Check sheet for the modelled part. Datum: model origin and axes. Units: mm. A direction names the side the tool comes from. Give positions to 0.01 mm unless a question says otherwise; leave off trailing zeros. Write each loop counter-clockwise with the first axis right and the second up, starting at its lowest first coordinate (ties: lowest second). Pieces come first, ordered by that corner, then holes. Notation, with made-up numbers: (23.25, -24.75) -> (69.25, -24.75) arc R19 ccw to (69.25, 3.25) -> close; hole circle Ø1 at (57.5, 22.25). An arc over 180 degrees is marked (long way). Use a Markdown table: item, result. Add a question column.
1. Set-up check for faces 4 (the flat face through (1.15, 8, 1)), 5 (the flat face through (4, -4, 0)): record each of +Z, -Z, +X, -X, +Y, -Y from which the full face is reachable in a straight line by a thin tool's end or side.
2. Cross-section at C-C (z = 3.3). Enter the section's corners in (x, y).
3. Cross-section at A-A (x = 0). Enter the section's corners in (y, z).
4. Gauge pin test, flat ends, axial feed: P1, Ø2, axis at y = 9, z = 2, coming from the +X side; P2, Ø2, axis at x = -10.5, z = 1.5, coming from the +Y side; P3, Ø1, axis at y = -14, z = 3, coming from the +X side; P4, Ø1.2, axis at y = -0.5, z = 1, coming from the -X side. Record the tip position at first contact, or that the pin passes through.
5. Scan lines: probe 1 along Y at (x, z) = (-0.5, 0.75); probe 2 along X at (y, z) = (-10.5, 1.35); probe 3 along Z at (x, y) = (-0.5, -1.5). Record each from-to range of solid material in increasing order. Write a range as [from, to].
6. Release check for a two-part mould opening along X. For faces 1 (the cylindrical face through (-3.848, -17.328, 0.863)), 2 (the flat face through (8, 1.15, 1)), 3 (the flat face through (0, 0, 4.25)) record: released by +X, released by -X, zero draft, split by the parting line, or undercut.
from build123d import *

# Parameters (mm, degrees)
SKETCH1_R           = 17.75
BOSS_EXTRUDE1_DEPTH = 4.25
CUT_EXTRUDE1_DEPTH  = 2.75
CHAMFER1_SIZE       = 2.5
CHAMFER1_SIZE2      = 1.443375673


with BuildPart() as part:
    # Sketch1 → Boss-Extrude1 (new body)
    with BuildSketch(Plane.XY):
        Circle(SKETCH1_R)
    extrude(amount=BOSS_EXTRUDE1_DEPTH)

    # Sketch2 → Cut-Extrude1 (cut)
    with BuildSketch(Plane(origin=(0, 0, 0), x_dir=(-1, 0, 0), z_dir=(0, 0, -1))):
        Polygon((-14.504482066, -1.15), (-14.504482066, 1.15), (-1.15, 1.15), (-1.15, 14.504482066), (1.15, 14.504482066), (1.15, 1.15), (14.504482066, 1.15), (14.504482066, -1.15), (1.15, -1.15), (1.15, -14.504482066), (-1.15, -14.504482066), (-1.15, -1.15), align=None)
    extrude(amount=-CUT_EXTRUDE1_DEPTH, mode=Mode.SUBTRACT)

    # Chamfer1
    chamfer1_edges = [part.edges().sort_by_distance(p)[0] for p in [
        (-17.75, 0, 4.25),
    ]]
    chamfer1_side = [part.faces().sort_by_distance(p)[0] for p in [
        (-17.75, 0, 2.125),
    ]]
    chamfer(chamfer1_edges, length=CHAMFER1_SIZE, length2=CHAMFER1_SIZE2, reference=chamfer1_side[0])


solid = part.part
Worked answers:
| question | item | result |
|---|---|---|
| 1 | face 4 | -Z |
| 1 | face 5 | -Z, +X, -X, +Y, -Y |
| 2 | outline | circle Ø33.71 at (0, 0) |
| 3 | outline | (-17.75, 0) -> (-14.5, 0) -> (-14.5, 2.75) -> (14.5, 2.75) -> (14.5, 0) -> (17.75, 0) -> (17.75, 1.75) -> (16.31, 4.25) -> (-16.31, 4.25) -> (-17.75, 1.75) -> close |
| 4 | P1 | stops at x = 15.83 |
| 4 | P2 | stops at y = 14.99 |
| 4 | P3 | stops at x = 10.53 |
| 4 | P4 | stops at x = -17.75 |
| 5 | probe 1 | y = [-17.74, -14.5], [14.5, 17.74] |
| 5 | probe 2 | x = [-14.31, -1.15], [1.15, 14.31] |
| 5 | probe 3 | z = [2.75, 4.25] |
| 6 | face 1 | split by the parting line |
| 6 | face 2 | undercut |
| 6 | face 3 | zero draft |
